Source: CAD feature listing. Evaluate the final solid. Frame: model axes, mm. A direction names the side the tool comes from. Round coordinates to 2 decimals unless told otherwise and drop trailing zeros. Write each loop counter-clockwise with the first axis right and the second up, starting at its lowest first coordinate (ties: lowest second). Pieces come first, ordered by that corner, then holes. Notation, with made-up numbers: M 20.5,-17.75 L 62.5,-17.75 A21 ccw 62.5,-10.75 Z; hole C -30.5,20.5 d2. An arc over 180 degrees is marked long. Put each result on its own line as item: value. Start each with the question number.
```python
from build123d import *

# Parameters (mm, degrees)
F0_R     = 2.25
F1_DEPTH = 12.5
F2_R     = 5


with BuildPart() as f1:
    # F0 (on Top) → F1 (new body, symmetric)
    with BuildSketch(Plane.XY):
        with BuildLine():
            Line((-12.5474100913, 30), (-30, 30))
            Line((-30, 30), (-30, 12.5474100913))
            Line((-30, 12.5474100913), (-27.25, 12.5474100913))
            ThreePointArc((-27.25, 12.5474100913), (-21.2132034356, 21.2132034356), (-12.5474100913, 27.25))
            Line((-12.5474100913, 27.25), (-12.5474100913, 30))
        make_face()
        with Locations((-25, 25)):
            Circle(F0_R, mode=Mode.SUBTRACT)
        with BuildLine():
            Line((-2.31e-08, 30), (-12.5474100913, 30))
            Line((-12.5474100913, 30), (-12.5474100913, 27.25))
            ThreePointArc((-12.5474100913, 27.25), (-6.4226163006, 29.3044365217), (-2.31e-08, 30))
        make_face()
        with BuildLine():
            Line((-27.25, 12.5474100913), (-30, 12.5474100913))
            Line((-30, 12.5474100913), (-30, 3.74e-08))
            ThreePointArc((-30, 3.74e-08), (-29.3044365202, 6.4226163076), (-27.25, 12.5474100913))
        make_face()
        with BuildLine():
            Line((12.5474100913, 30), (-2.31e-08, 30))
            ThreePointArc((-2.31e-08, 30), (6.422616278, 29.3044365267), (12.5474100913, 27.25))
            Line((12.5474100913, 27.25), (12.5474100913, 30))
        make_face()
        with BuildLine():
            ThreePointArc((12.5474100913, 27.25), (6.422616278, 29.3044365267), (-2.31e-08, 30))
            ThreePointArc((-2.31e-08, 30), (-6.4226163006, 29.3044365217), (-12.5474100913, 27.25))
            Line((-12.5474100913, 27.25), (12.5474100913, 27.25))
        make_face()
        with BuildLine():
            ThreePointArc((-27.25, -12.5474100913), (-29.3044365282, -6.4226162711), (-30, 3.74e-08))
            Line((-30, 3.74e-08), (-30, -12.5474100913))
            Line((-30, -12.5474100913), (-27.25, -12.5474100913))
        make_face()
        with BuildLine():
            ThreePointArc((-27.25, 12.5474100913), (-29.3044365202, 6.4226163076), (-30, 3.74e-08))
            ThreePointArc((-30, 3.74e-08), (-29.3044365282, -6.4226162711), (-27.25, -12.5474100913))
            Line((-27.25, -12.5474100913), (-27.25, 12.5474100913))
        make_face()
        with BuildLine():
            Line((30, 30), (12.5474100913, 30))
            Line((12.5474100913, 30), (12.5474100913, 27.25))
            ThreePointArc((12.5474100913, 27.25), (21.2132034356, 21.2132034356), (27.25, 12.5474100913))
            Line((27.25, 12.5474100913), (30, 12.5474100913))
            Line((30, 12.5474100913), (30, 30))
        make_face()
        with Locations((25, 25)):
            Circle(F0_R, mode=Mode.SUBTRACT)
        with BuildLine():
            Line((-27.25, -12.5474100913), (-30, -12.5474100913))
            Line((-30, -12.5474100913), (-30, -30))
            Line((-30, -30), (-12.5474100913, -30))
            Line((-12.5474100913, -30), (-12.5474100913, -27.25))
            ThreePointArc((-12.5474100913, -27.25), (-21.2132034356, -21.2132034356), (-27.25, -12.5474100913))
        make_face()
        with Locations((-25, -25)):
            Circle(F0_R, mode=Mode.SUBTRACT)
        with BuildLine():
            Line((30, 12.5474100913), (27.25, 12.5474100913))
            ThreePointArc((27.25, 12.5474100913), (29.3044365242, 6.4226162893), (30, 0))
            Line((30, 0), (30, 12.5474100913))
        make_face()
        with BuildLine():
            ThreePointArc((30, 0), (29.3044365242, 6.4226162893), (27.25, 12.5474100913))
            Line((27.25, 12.5474100913), (27.25, -12.5474100913))
            ThreePointArc((27.25, -12.5474100913), (29.3044365242, -6.4226162893), (30, 0))
        make_face()
        with BuildLine():
            Line((12.5474100913, -27.25), (-12.5474100913, -27.25))
            ThreePointArc((-12.5474100913, -27.25), (-6.4226162893, -29.3044365242), (0, -30))
            ThreePointArc((0, -30), (6.4226162893, -29.3044365242), (12.5474100913, -27.25))
        make_face()
        with BuildLine():
            ThreePointArc((0, -30), (-6.4226162893, -29.3044365242), (-12.5474100913, -27.25))
            Line((-12.5474100913, -27.25), (-12.5474100913, -30))
            Line((-12.5474100913, -30), (0, -30))
        make_face()
        with BuildLine():
            Line((30, -12.5474100913), (30, 0))
            ThreePointArc((30, 0), (29.3044365242, -6.4226162893), (27.25, -12.5474100913))
            Line((27.25, -12.5474100913), (30, -12.5474100913))
        make_face()
        with BuildLine():
            Line((30, -12.5474100913), (27.25, -12.5474100913))
            ThreePointArc((27.25, -12.5474100913), (21.2132034356, -21.2132034356), (12.5474100913, -27.25))
            Line((12.5474100913, -27.25), (12.5474100913, -30))
            Line((12.5474100913, -30), (30, -30))
            Line((30, -30), (30, -12.5474100913))
        make_face()
        with Locations((25, -25)):
            Circle(F0_R, mode=Mode.SUBTRACT)
        with BuildLine():
            ThreePointArc((12.5474100913, -27.25), (6.4226162893, -29.3044365242), (0, -30))
            Line((0, -30), (12.5474100913, -30))
            Line((12.5474100913, -30), (12.5474100913, -27.25))
        make_face()
    extrude(amount=F1_DEPTH, both=True)

    # F2
    f2_edges = [f1.edges().sort_by_distance(p)[0] for p in [
        (-30, 30, 0),
        (30, -30, 0),
        (30, 30, 0),
        (-30, -30, 0),
    ]]
    fillet(f2_edges, radius=F2_R)


solid = f1.part
```
(1) Pull-direction query (X, two-part tool) for faces 3 (the cylindrical face through (-28, -29, 0)), 4 (the cylindrical face through (28, -29, 0)), 5 (the cylindrical face through (21.318, -21.108, 0.175)); classes: +X half, -X half, draft (parallel to the pull), parting line (faces both ways), or undercut.
(2) Contact query for flat-ended pins moving along their axis: P1, Ø5, axis at x = 25, y = 25, coming from the -Z side; P2, Ø2.5, axis at x = -25, y = 25, coming from the -Z side (3 decimals). Output: stop coordinate, or through.
(3) Section query C-C (z = -7). Return loops of the section in (x, y), and give its area (3 significant figures).
(4) Section query A-A (y = -2.5). Return loops of the section in (x, z).
(5) Access query for faces 1 (the flat face through (0, -27.25, 0)), 2 (the flat face through (0, -30, 0)). Directions: +Z, -Z, +X, -X, +Y, -Y. A direction counts if a zero-diameter tool reaches every point of the face in a straight line with its end or side. Return the directions, or none.
(6) Section query D-D (y = 23.5). Return loops of the section in (x, z).
(7) Ray query, line 1 along Y through (x, z) = (-25, 2); line 2 along X through (y, z) = (-6.5, 1.5). Return the intervals inside material, ascending.
Entries:
1. face 3: -X half
1. face 4: +X half
1. face 5: undercut
2. P1: z = -12.5
2. P2: through
3. outline: M -30,-25 A5 ccw -25,-30 L 25,-30 A5 ccw 30,-25 L 30,25 A5 ccw 25,30 L -25,30 A5 ccw -30,25 Z; hole C -25,-25 d4.5; hole M -27.25,-12.55 A30 ccw -12.55,-27.25 L 12.55,-27.25 A30 ccw 27.25,-12.55 L 27.25,12.55 A30 ccw 12.55,27.25 L -12.55,27.25 A30 ccw -27.25,12.55 Z; hole C -25,25 d4.5; hole C 25,-25 d4.5; hole C 25,25 d4.5
3. area: 873 mm2
4. outline: M -30,-12.5 L -27.25,-12.5 L -27.25,12.5 L -30,12.5 Z; M 27.25,-12.5 L 30,-12.5 L 30,12.5 L 27.25,12.5 Z
5. face 1: +Z, -Z
5. face 2: +Z, -Z, +X, -X, -Y
6. outline: M -30,-12.5 L -26.68,-12.5 L -26.68,12.5 L -30,12.5 Z; M -23.32,-12.5 L -18.65,-12.5 L -18.65,12.5 L -23.32,12.5 Z; M 18.65,-12.5 L 23.32,-12.5 L 23.32,12.5 L 18.65,12.5 Z; M 26.68,-12.5 L 30,-12.5 L 30,12.5 L 26.68,12.5 Z
7. line 1: -30 to -27.25, -22.75 to -16.58, 16.58 to 22.75, 27.25 to 30
7. line 2: -30 to -27.25, 27.25 to 30
